```python
from build123d import *

# Parameters (mm, degrees)
SKETCH1_W           = 120
SKETCH1_H           = 220
SKETCH1_R           = 6
SKETCH1_R_2         = 3.5
BOSS_EXTRUDE1_DEPTH = 10


with BuildPart() as part:
    # Sketch1 → Boss-Extrude1 (new body)
    with BuildSketch(Plane.XY):
        with Locations((0, -94.764397906)):
            Rectangle(SKETCH1_W, SKETCH1_H)
        with Locations((0, -14.764397906)):
            Circle(SKETCH1_R, mode=Mode.SUBTRACT)
        with Locations((24, -14.764397906)):
            Circle(SKETCH1_R_2, mode=Mode.SUBTRACT)
        with Locations(Location((-24, -14.764397906, 0), (0, 0, 180))):
            Circle(SKETCH1_R_2, mode=Mode.SUBTRACT)
        with BuildLine():
            Line((4, -114.764397906), (4, -134.764397906))
            ThreePointArc((4, -134.764397906), (0, -138.764397906), (-4, -134.764397906))
            Line((-4, -134.764397906), (-4, -114.764397906))
            ThreePointArc((-4, -114.764397906), (0, -110.764397906), (4, -114.764397906))
        make_face(mode=Mode.SUBTRACT)
        with BuildLine():
            Line((23.15, -114.764397906), (23.15, -134.764397906))
            ThreePointArc((23.15, -134.764397906), (20.65, -137.264397906), (18.15, -134.764397906))
            Line((18.15, -134.764397906), (18.15, -114.764397906))
            ThreePointArc((18.15, -114.764397906), (20.65, -112.264397906), (23.15, -114.764397906))
        make_face(mode=Mode.SUBTRACT)
        with BuildLine():
            Line((-23.15, -114.764397906), (-23.15, -134.764397906))
            ThreePointArc((-23.15, -134.764397906), (-20.65, -137.264397906), (-18.15, -134.764397906))
            Line((-18.15, -134.764397906), (-18.15, -114.764397906))
            ThreePointArc((-18.15, -114.764397906), (-20.65, -112.264397906), (-23.15, -114.764397906))
        make_face(mode=Mode.SUBTRACT)
        with BuildLine():
            Line((-23.15, -176.064397906), (-23.15, -156.064397906))
            ThreePointArc((-23.15, -156.064397906), (-20.65, -153.564397906), (-18.15, -156.064397906))
            Line((-18.15, -156.064397906), (-18.15, -176.064397906))
            ThreePointArc((-18.15, -176.064397906), (-20.65, -178.564397906), (-23.15, -176.064397906))
        make_face(mode=Mode.SUBTRACT)
        with BuildLine():
            Line((23.15, -176.064397906), (23.15, -156.064397906))
            ThreePointArc((23.15, -156.064397906), (20.65, -153.564397906), (18.15, -156.064397906))
            Line((18.15, -156.064397906), (18.15, -176.064397906))
            ThreePointArc((18.15, -176.064397906), (20.65, -178.564397906), (23.15, -176.064397906))
        make_face(mode=Mode.SUBTRACT)
    extrude(amount=BOSS_EXTRUDE1_DEPTH)


solid = part.part
```
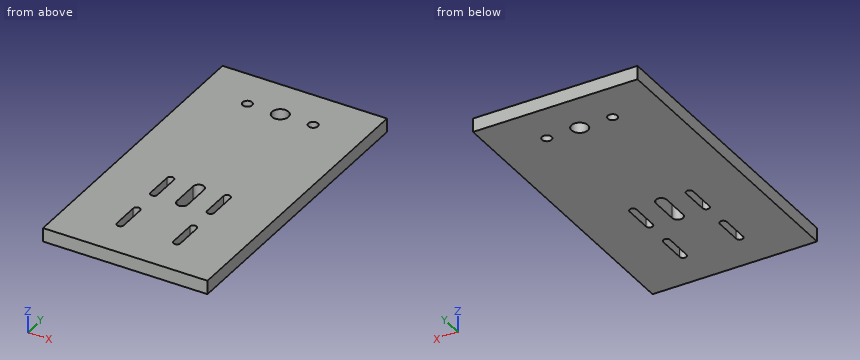
Input: part model. Units: mm. Frame: model coordinates. Round coordinates to 2 decimals unless told otherwise and drop trailing zeros. Order: outer loops, then holes, each group sorted by start corner. A loop starts at its lowest first (then second) coordinate and runs counter-clockwise, first axis right, second up. Notation, with made-up numbers: (59.5, 36) - (74.5, 36) arc R28 cw to (74.5, 54) - close; hole circle Ø11 at (10.5, 28.25). An arc over 180 degrees is marked (long way). One line per question, with ' | ' between items. Start each with the question number.
1) Ray query, probe 1 along X at (y, z) = (-163.5, 9); probe 2 along X at (y, z) = (-116.5, 1.5); probe 3 along Y at (x, z) = (24, 8.25). Return the intervals inside material, ascending.
2) Contact query for a flat-ended pin moving along its axis: P1, Ø5.5, axis at x = -24, y = -14.76, coming from the -Z side. Output: stop coordinate, or through.
3) Cut plane A-A, the plane x = 0. Return the cut outline in (y, z), then the cut area to 3 significant figures.
4) Cut plane B-B, the plane z = 7. Give the number of separate pieces and of enclosed holes in the cut face, then the cut area to 3 significant figures.
Worked out:
1) probe 1: x = -60 to -23.15, -18.15 to 18.15, 23.15 to 60 | probe 2: x = -60 to -23.15, -18.15 to -4, 4 to 18.15, 23.15 to 60 | probe 3: y = -204.76 to -18.26, -11.26 to 15.24
2) P1: passes through
3) outline: (-204.76, 0) - (-138.76, 0) - (-138.76, 10) - (-204.76, 10) - close; (-110.76, 0) - (-20.76, 0) - (-20.76, 10) - (-110.76, 10) - close; (-8.76, 0) - (15.24, 0) - (15.24, 10) - (-8.76, 10) - close | area: 1,800 mm^2
4) separate pieces: 1 | enclosed holes: 8 | area: 25,500 mm^2
